Can you work these out from the model? Positions are in its coordinate system, mm. Face numbers are marked on the shaded views. A direction names the side the tool comes from. Round coordinates to 2 decimals unless told otherwise and drop trailing zeros. Order: outer loops, then holes, each group sorted by start corner. A loop starts at its lowest first (then second) coordinate and runs counter-clockwise, first axis right, second up.
Q1. Will these pins go through, and if not, where does the flat tip stop? P1, Ø8, axis at x = 35, y = 35, coming from the +Z side; P2, Ø5, axis at y = 27, z = -24, coming from the +X side; P3, Ø6, axis at y = 43, z = -4, coming from the +X side.
Q2. If we section it at B-B (z = 0): Please give me the cut outline in (x, y), plus the area to 3 significant figures.
Q3. We'd pull the mould along Y, two halves only. Please class the marked faces 1, 2, 3 and 4: pulls with the +Y half, pulls with the -Y half, needs draft (parallel to the pull), parting line crosses it, or undercut.
Q4. For the marked faces 5 and 6, which set-ups out of +Z, -Z, +X, -X, +Y, -Y let a thin tool reach every point of the face, with its end or its side?
Q5. If I drill on line 1 (Y direction, x = -89, z = 32); line 2 (Z direction, x = 0, y = 59.5); line 3 (X direction, y = 9, z = 6.5), over which ranges is the centre line in solid material (lowest first)?
Q6. If we section it at D-D (x = 40): Please give me the cut outline in (y, z).
Q7. If we section it at C-C (y = 22): Please give me the cut outline in (x, z).
Q8. If we section it at A-A (x = 0): Please give me the cut outline in (y, z).
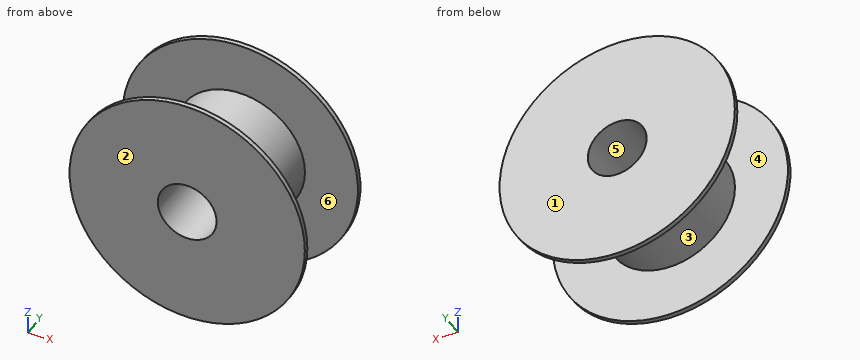
from build123d import *

# Parameters (mm, degrees)
F0_R     = 100
F1_DEPTH = 4
F2_R     = 55
F3_DEPTH = 84
F4_R     = 100
F4_R_2   = 55
F5_DEPTH = 4
F6_R     = 25
F7_DEPTH = 88


with BuildPart() as f1:
    # F0 (on Front) → F1 (new body)
    with BuildSketch(Plane.XZ):
        Circle(F0_R)
    extrude(amount=F1_DEPTH)

    # F2 (on face) → F3 (join)
    with BuildSketch(Plane(origin=(0, 0, 0), x_dir=(-1, 0, 0), z_dir=(0, 1, 0))):
        Circle(F2_R)
    extrude(amount=F3_DEPTH)

    # F4 (on face) → F5 (join)
    with BuildSketch(Plane(origin=(0, 84, 0), x_dir=(-1, 0, 0), z_dir=(0, 1, 0))):
        Circle(F4_R)
        Circle(F4_R_2, mode=Mode.SUBTRACT)
    extrude(amount=-F5_DEPTH)

    # F6 (on face) → F7 (cut, through all)
    with BuildSketch(Plane(origin=(0, 84, 0), x_dir=(-1, 0, 0), z_dir=(0, 1, 0))):
        Circle(F6_R)
    extrude(amount=-F7_DEPTH, mode=Mode.SUBTRACT)


solid = f1.part
Solution:
1. P1: stops at z = 45.43
1. P2: stops at x = 50.62
1. P3: stops at x = 54.99
2. outline: (-100, -4) - (-25, -4) - (-25, 84) - (-100, 84) - (-100, 80) - (-55, 80) - (-55, 0) - (-100, 0) - close; (25, -4) - (100, -4) - (100, 0) - (55, 0) - (55, 80) - (100, 80) - (100, 84) - (25, 84) - close
2. area: 6,000 mm2
3. face 1: pulls with the +Y half
3. face 2: pulls with the -Y half
3. face 3: undercut
3. face 4: undercut
4. face 5: +Y, -Y
4. face 6: none
5. line 1: y = -4 to 0, 80 to 84
5. line 2: z = -55 to -25, 25 to 55
5. line 3: x = -54.61 to -24.14, 24.14 to 54.61
6. outline: (-4, -91.65) - (0, -91.65) - (0, -37.75) - (80, -37.75) - (80, -91.65) - (84, -91.65) - (84, 91.65) - (80, 91.65) - (80, 37.75) - (0, 37.75) - (0, 91.65) - (-4, 91.65) - close
7. outline: circle Ø110 at (0, 0); hole circle Ø50 at (0, 0)
8. outline: (-4, -100) - (0, -100) - (0, -55) - (80, -55) - (80, -100) - (84, -100) - (84, -25) - (-4, -25) - close; (-4, 25) - (84, 25) - (84, 100) - (80, 100) - (80, 55) - (0, 55) - (0, 100) - (-4, 100) - close
